Input: part model. Units: mm. Frame: model coordinates. Give positions to 0.01 mm unless a question says otherwise; leave off trailing zeros. Write each loop counter-clockwise with the first axis right and the second up, starting at its lowest first coordinate (ties: lowest second). Pieces come first, ordered by that corner, then holes. Notation, with made-up numbers: (70, 89) -> (79, 89) arc R34 cw to (79, 122) -> close; hole circle Ø4 at (-10, -2.5). An arc over 180 degrees is marked (long way). Return JSON: item names as keys, results as strings. Group by question number.
Item 1: Section A-A, the plane x = 215.5. Return loops of the section in (y, z), then the cut area to 3 significant figures.
Item 2: Pin query (flat end, axial travel): P1, Ø2.5, axis at x = 215.75, y = 241.95, coming from the +Z side; P2, Ø1.5, axis at y = 250, z = 0.5, coming from the -X side. Return the tip coordinate at first contact, or that it passes through.
Item 3: Section D-D, the plane x = 225.25. Return loops of the section in (y, z).
Item 4: Section B-B, the plane z = 2.1. Return loops of the section in (x, y).
Item 5: Mould query, pull axis X, two halves, no side actions, for faces 1 (the face through (224.42, 240.49, 1.48)), 2 (the face through (210.36, 254.91, 1.48)), 3 (the face through (221.136, 228.995, 1.479)). Classes: released by +X, released by -X, zero draft, split by the parting line, or undercut.
Item 6: Line query: line 1 (X direction, y = 243, z = 2.6); line 2 (X direction, y = 241, z = 0.3); line 3 (Y direction, x = 207.75, z = 1.5). Output: solid intervals per line, ascending. Write a range as [from, to].
Item 7: Section C-C, the plane y = 233.75. Return loops of the section in (x, z).
from build123d import *

# Parameters (mm, degrees)
MODEL_R                 = 1.5
SALIENTE_EXTRUIR1_DEPTH = 3


with BuildPart() as part:
    # Model → Saliente-Extruir1 (new body)
    with BuildSketch(Plane.XY):
        Polygon((219.837619938, 228.457019993), (211.657995889, 228.457019993), (209.097335717, 229.517680165), (203.313468085, 235.301547797), (202.252807913, 237.862207969), (202.252807913, 246.041832017), (203.313468085, 248.602492189), (209.097335717, 254.386359821), (211.657995889, 255.447019993), (219.837619938, 255.447019993), (222.39828011, 254.386359821), (228.182147742, 248.602492189), (229.242807914, 246.041832017), (229.242807914, 237.862207969), (228.182147742, 235.301547797), (222.39828011, 229.517680165), align=None)
        with Locations((215.747807914, 241.952019993)):
            Circle(MODEL_R, mode=Mode.SUBTRACT)
        with Locations((215.747807914, 232.952019993)):
            Circle(MODEL_R, mode=Mode.SUBTRACT)
        with Locations((215.747807914, 250.952019993)):
            Circle(MODEL_R, mode=Mode.SUBTRACT)
        with Locations((224.747807913, 241.952019993)):
            Circle(MODEL_R, mode=Mode.SUBTRACT)
        with Locations((206.747807913, 241.952019993)):
            Circle(MODEL_R, mode=Mode.SUBTRACT)
    extrude(amount=SALIENTE_EXTRUIR1_DEPTH)


solid = part.part
Answer below:
{
 "1": {"outline": "(228.46, 0) -> (231.47, 0) -> (231.47, 3) -> (228.46, 3) -> close; (234.43, 0) -> (240.47, 0) -> (240.47, 3) -> (234.43, 3) -> close; (243.43, 0) -> (249.47, 0) -> (249.47, 3) -> (243.43, 3) -> close; (252.43, 0) -> (255.45, 0) -> (255.45, 3) -> (252.43, 3) -> close", "area": "54.3 mm2"},
 "2": {"P1": "passes through", "P2": "stops at x = 203.96"},
 "3": {"outline": "(232.37, 0) -> (240.54, 0) -> (240.54, 3) -> (232.37, 3) -> close; (243.37, 0) -> (251.53, 0) -> (251.53, 3) -> (243.37, 3) -> close"},
 "4": {"outline": "(202.25, 237.86) -> (203.31, 235.3) -> (209.1, 229.52) -> (211.66, 228.46) -> (219.84, 228.46) -> (222.4, 229.52) -> (228.18, 235.3) -> (229.24, 237.86) -> (229.24, 246.04) -> (228.18, 248.6) -> (222.4, 254.39) -> (219.84, 255.45) -> (211.66, 255.45) -> (209.1, 254.39) -> (203.31, 248.6) -> (202.25, 246.04) -> close; hole circle Ø3 at (206.75, 241.95); hole circle Ø3 at (215.75, 232.95); hole circle Ø3 at (215.75, 241.95); hole circle Ø3 at (215.75, 250.95); hole circle Ø3 at (224.75, 241.95)"},
 "5": {"face 1": "undercut", "face 2": "released by -X", "face 3": "released by +X"},
 "6": {"line 1": "x = [202.25, 205.67], [207.82, 214.67], [216.82, 223.67], [225.82, 229.24]", "line 2": "x = [202.25, 205.59], [207.91, 214.59], [216.91, 223.59], [225.91, 229.24]", "line 3": "y = [230.87, 240.84], [243.07, 253.04]"},
 "7": {"outline": "(204.87, 0) -> (214.48, 0) -> (214.48, 3) -> (204.87, 3) -> close; (217.02, 0) -> (226.63, 0) -> (226.63, 3) -> (217.02, 3) -> close"}
}
